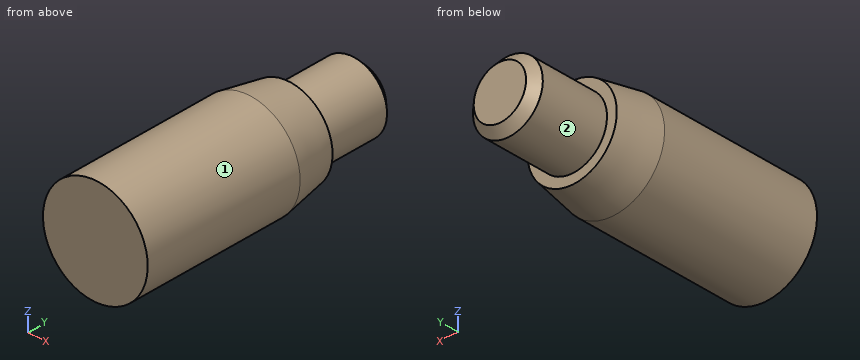
```python
from build123d import *

# Parameters (mm, degrees)
CHANFREIN1_SIZE = 1


with BuildPart() as part:
    # Esquisse1 → Révolution1 (revolve)
    with BuildSketch(Plane.XY, mode=Mode.PRIVATE) as r_volution1_sk:
        Polygon((0, 0), (6, 0), (6, 19), (5.118365096, 24), (4, 24), (4, 33), (0, 33), align=None)
    revolve(r_volution1_sk.sketch.rotate(Axis((0, 0, 0), (0, 1, 0)), 90), axis=Axis((0, 0, 0), (0, 1, 0)))

    # Chanfrein1
    chanfrein1_edges = [part.edges().sort_by_distance(p)[0] for p in [
        (0, 33, 4),
    ]]
    chamfer(chanfrein1_edges, length=CHANFREIN1_SIZE)


solid = part.part
```
Can you work these out from the model? Positions are in its coordinate system, mm. Face numbers are marked on the shaded views. A direction names the side the tool comes from. Coordinates: 2 decimals unless noted, no trailing zeros. Loops run counter-clockwise (first coordinate to the right, second up) from the corner with the lowest first, then second, coordinate; pieces in that order, holes last.
1) Imagine slicing it at B-B on z = 0. List the corners of the cut face in (x, y) for me, plus the area to 3 significant figures.
2) Which directions (+Z, -Z, +X, -X, +Y, -Y) give clear straight access to the entire face, cutting with the end or side of a thin tool? Please do the marked faces 1 and 2.
3) Imagine slicing it at A-A on x = 0. List the corners of the cut face in (y, z) for me, plus the area to 3 significant figures.
4) I need wall thicknesses on probe 1 along Y at (x, z) = (0.25, 5); probe 2 along X at (y, z) = (31, -0.25); probe 3 along Y at (x, z) = (-3.5, 0.5). Which ranges of each line are inside material? Lowest first, please.
5) For pin 1 (2 mm diameter, centred on x = 3, y = 5, fed in from -Z); pin 2 (2 mm diameter, centred on y = 12, z = -2.5, fed in from +X); pin 3 (6 mm diameter, centred on y = 13.5, z = -3.5, fed in from -X), each with a flat end and sliding along its axis, tell me the tip position at first contact or that it passes through.
6) Imagine slicing it at C-C on y = 7. List the corners of the cut face in (x, z) for me, plus the area to 3 significant figures.
Completed:
1. outline: (-6, 0) - (6, 0) - (6, 19) - (5.12, 24) - (4, 24) - (4, 32) - (3, 33) - (-3, 33) - (-4, 32) - (-4, 24) - (-5.12, 24) - (-6, 19) - close
1. area: 355 mm2
2. face 1: +Y, -Y
2. face 2: +Y
3. outline: (0, -6) - (19, -6) - (24, -5.12) - (24, -4) - (32, -4) - (33, -3) - (33, 3) - (32, 4) - (24, 4) - (24, 5.12) - (19, 6) - (0, 6) - close
3. area: 355 mm2
4. probe 1: y = 0 to 24
4. probe 2: x = -3.99 to 3.99
4. probe 3: y = 0 to 32.46
5. pin 1: stops at z = -5.66
5. pin 2: stops at x = 5.81
5. pin 3: stops at x = -5.98
6. outline: circle Ø12 at (0, 0)
6. area: 113 mm2
